```python
from build123d import *

# Parameters (mm, degrees)
BOSS_EXTRUDE1_DEPTH         = 4.7625
F_1_4_0_25_DIAMETER_HOLE2_D = 6.35
F_4_0MM_DOWEL_HOLE1_D       = 4
F_1_4_20_TAPPED_HOLE1_D     = 5.1054


with BuildPart() as part:
    # Sketch1 → Boss-Extrude1 (new body)
    with BuildSketch(Plane.XY):
        with BuildLine():
            Line((-132.526798161, -26.601306725), (-2.419218956, 5.838156153))
            ThreePointArc((-2.419218956, 5.838156153), (0, 6.13519889), (2.419218956, 5.838156153))
            Line((2.419218956, 5.838156153), (132.526798161, -26.601306725))
            ThreePointArc((132.526798161, -26.601306725), (138.679252212, -31.153883239), (139.810536468, -38.723482944))
            Line((139.810536468, -38.723482944), (125.295222732, -96.941226521))
            ThreePointArc((125.295222732, -96.941226521), (120.742646218, -103.093680572), (113.173046513, -104.224964827))
            Line((113.173046513, -104.224964827), (2.419218956, -76.610934195))
            ThreePointArc((2.419218956, -76.610934195), (0, -76.313891458), (-2.419218956, -76.610934195))
            Line((-2.419218956, -76.610934195), (-113.173046513, -104.224964827))
            ThreePointArc((-113.173046513, -104.224964827), (-120.742646218, -103.093680572), (-125.295222732, -96.941226521))
            Line((-125.295222732, -96.941226521), (-139.810536468, -38.723482944))
            ThreePointArc((-139.810536468, -38.723482944), (-138.679252212, -31.153883239), (-132.526798161, -26.601306725))
        make_face()
    extrude(amount=-BOSS_EXTRUDE1_DEPTH)

    # 1/4 (0.25) Diameter Hole2 (through all)
    with Locations(Plane.XY):
        with Locations((-74.335136024, -53.317040996), (74.335136024, -53.317040996)):
            Hole(F_1_4_0_25_DIAMETER_HOLE2_D / 2)

    # Ø4.0mm Dowel Hole1 (through all)
    with Locations(Plane.XY):
        with Locations((-110.721225759, -62.389112081), (-37.949046288, -44.244969911), (37.949046288, -44.244969911), (110.721225759, -62.389112081)):
            Hole(F_4_0MM_DOWEL_HOLE1_D / 2)

    # 1/4-20 Tapped Hole1 (through all)
    with Locations(Plane.XY):
        with Locations((-7.366, -20.569560235), (-7.366, -58.669560235)):
            Hole(F_1_4_20_TAPPED_HOLE1_D / 2)


solid = part.part
```
Geometry: final body of the model. Coordinates: model frame, mm. A direction names the side the tool comes from. Coordinates: 2 decimals unless noted, no trailing zeros. Order: outer loops, then holes, each group sorted by start corner. A loop starts at its lowest first (then second) coordinate and runs counter-clockwise, first axis right, second up. Notation, with made-up numbers: (43.5, 34.25) - (49.5, 34.25) arc R21 cw to (49.5, 65.25) - close; hole circle Ø4 at (34.25, -20.75). An arc over 180 degrees is marked (long way). Return JSON: item names as keys, results as strings. Group by question number.
1. Pull-direction query (X, two-part tool) for faces 3 (the face through (-68.384, -10.609, -2.348)), 4 (the face through (-0.034, 6.135, -2.348)), 5 (the face through (-71.995, -51.171, -2.415)); classes: pulls with the +X half, pulls with the -X half, needs draft (parallel to the pull), parting line crosses it, or undercut.
2. Cut plane D-D (y = -8). Output: boundary loops of the cut face in (x, z), plus the area to 3 significant figures.
3. Pin query (flat end, axial travel): pin 1 (1.5 mm diameter, centred on y = -50, z = -3, fed in from -X). Return the tip coordinate at first contact, or that it passes through.
4. Cut plane A-A (y = -79.5). Output: boundary loops of the cut face in (x, z).
5. Material intervals for line 1 along Y through (x, z) = (-9, -1.7); line 2 along X through (y, z) = (-62, -2.4); line 3 along X through (y, z) = (-43.5, -3.7), sorted ascending. Write a range as [from, to].
6. Cut plane B-B (z = -2.2). Count the separate pieces of the cut face and the enclosed holes in it, plus the area to 3 significant figures.
7. Set-up query: faces 1 (the face through (58.57, -90.61, -2.35)), 2 (the face through (66.562, -10.154, -2.348)). Return all of +Z, -Z, +X, -X, +Y, -Y with unobstructed straight access to the full face (end or side cutting, diameter ignored); none if empty.
8. Cut plane C-C (x = -20.5). Output: boundary loops of the cut face in (y, z), plus the area to 3 significant figures.
Resolved:
{
 "1": {"face 3": "pulls with the -X half", "face 4": "parting line crosses it", "face 5": "undercut"},
 "2": {"outline": "(-57.92, -4.76) - (57.92, -4.76) - (57.92, 0) - (-57.92, 0) - close", "area": "552 mm²"},
 "3": {"pin 1": "stops at x = -137.19"},
 "4": {"outline": "(-129.64, -4.76) - (-14.01, -4.76) - (-14.01, 0) - (-129.64, 0) - close; (14.01, -4.76) - (129.64, -4.76) - (129.64, 0) - (14.01, 0) - close"},
 "5": {"line 1": "y = [-78.25, -60.63], [-56.71, -22.53], [-18.61, 4.2]", "line 2": "x = [-134.01, -112.68], [-108.76, 108.76], [112.68, 134.01]", "line 3": "x = [-138.62, -39.81], [-36.09, 36.09], [39.81, 138.62]"},
 "6": {"separate pieces": "1", "enclosed holes": "8", "area": "21,600 mm²"},
 "7": {"face 1": "+Z, -Z, -Y", "face 2": "+Z, -Z, +X, +Y"},
 "8": {"outline": "(-81.12, -4.76) - (1.33, -4.76) - (1.33, 0) - (-81.12, 0) - close", "area": "393 mm²"}
}
